```python
from build123d import *

# Parameters (mm, degrees)
F0_R     = 1.7272
F0_R_2   = 3.2639
F0_R_3   = 2.4003
F1_DEPTH = 99.06
F2_DEPTH = 88.9
F3_DEPTH = 25.4
F4_DEPTH = 99.061
F5_R     = 1.7272
F6_DEPTH = 5.08
F7_DEPTH = 15.24
F5_R_2   = 1.5875
F8_DEPTH = 19.6383854826


with BuildPart() as f1:
    # F0 (on Front) → F1 (new body)
    with BuildSketch(Plane.XZ):
        with BuildLine():
            Line((-9.525, -12.7), (9.525, -12.7))
            ThreePointArc((9.525, -12.7), (0, 15.875), (-9.525, -12.7))
        make_face()
        with Locations((-9.525, -1.905)):
            Circle(F0_R, mode=Mode.SUBTRACT)
        with Locations((9.525, -1.905)):
            Circle(F0_R, mode=Mode.SUBTRACT)
        with Locations((0, 8.7377419695)):
            Circle(F0_R_2, mode=Mode.SUBTRACT)
        with Locations((0, 8.7377419695)):
            Circle(F0_R_2)
        with Locations((0, 8.7377419695)):
            Circle(F0_R_3, mode=Mode.SUBTRACT)
        with Locations((-9.525, -1.905)):
            Circle(F0_R)
        with Locations((9.525, -1.905)):
            Circle(F0_R)
    extrude(amount=-F1_DEPTH)

    # F0 (on Front) → F2 (cut, through all)
    with BuildSketch(Plane.XZ):
        with Locations((0, 8.7377419695)):
            Circle(F0_R_2)
        with Locations((0, 8.7377419695)):
            Circle(F0_R_3, mode=Mode.SUBTRACT)
    extrude(amount=-F2_DEPTH, mode=Mode.SUBTRACT)

    # F0 (on Front) → F3 (cut)
    with BuildSketch(Plane.XZ):
        with Locations((-9.525, -1.905)):
            Circle(F0_R)
        with Locations((9.525, -1.905)):
            Circle(F0_R)
    extrude(amount=-F3_DEPTH, mode=Mode.SUBTRACT)

    # F0 (on Front) → F4 (cut, through all)
    with BuildSketch(Plane.XZ):
        with Locations((0, 8.7377419695)):
            Circle(F0_R_3)
    extrude(amount=-F4_DEPTH, mode=Mode.SUBTRACT)

    # F5 (on face) → F6 (cut)
    with BuildSketch(Plane(origin=(0, 0, -12.7), x_dir=(1, 0, 0), z_dir=(0, 0, -1))):
        with BuildLine():
            Line((-9.525, -84.5499397641), (-9.525, -8.5156602359))
            ThreePointArc((-9.525, -8.5156602359), (-17.1876576863, -11.3104638467), (-24.1058971733, -15.6307893484))
            Line((-24.1058971733, -15.6307893484), (-24.1058971733, -77.4348106516))
            ThreePointArc((-24.1058971733, -77.4348106516), (-17.1876576863, -81.7551361533), (-9.525, -84.5499397641))
        make_face()
        with BuildLine():
            Line((9.525, -84.5499397641), (9.525, -8.5156602359))
            ThreePointArc((9.525, -8.5156602359), (0, -7.3406), (-9.525, -8.5156602359))
            Line((-9.525, -8.5156602359), (-9.525, -84.5499397641))
            ThreePointArc((-9.525, -84.5499397641), (0, -85.725), (9.525, -84.5499397641))
        make_face()
        with Locations((0, -46.5328)):
            Circle(F5_R, mode=Mode.SUBTRACT)
        with BuildLine():
            ThreePointArc((19.2613247782, -12.4002655405), (14.5236243119, -10.1309748028), (9.525, -8.5156602359))
            Line((9.525, -8.5156602359), (9.525, -84.5499397641))
            ThreePointArc((9.525, -84.5499397641), (14.5236243119, -82.9346251972), (19.2613247782, -80.6653344595))
            Line((19.2613247782, -80.6653344595), (19.2613247782, -12.4002655405))
        make_face()
        with BuildLine():
            ThreePointArc((19.2613247782, -87.8013515693), (14.4855288925, -89.7098938525), (9.525, -91.067801469))
            Line((9.525, -91.067801469), (9.525, -99.06))
            Line((9.525, -99.06), (19.2613247782, -99.06))
            Line((19.2613247782, -99.06), (19.2613247782, -87.8013515693))
        make_face()
        with BuildLine():
            Line((9.525, -99.06), (9.525, -91.067801469))
            ThreePointArc((9.525, -91.067801469), (0, -92.075), (-9.525, -91.067801469))
            Line((-9.525, -91.067801469), (-9.525, -99.06))
            Line((-9.525, -99.06), (9.525, -99.06))
        make_face()
        with BuildLine():
            Line((-9.525, -99.06), (-9.525, -91.067801469))
            ThreePointArc((-9.525, -91.067801469), (-17.0718789618, -88.7541563206), (-24.1058971733, -85.1721284402))
            Line((-24.1058971733, -85.1721284402), (-24.1058971733, -99.06))
            Line((-24.1058971733, -99.06), (-9.525, -99.06))
        make_face()
        with BuildLine():
            Line((9.525, 0), (9.525, -1.997798531))
            ThreePointArc((9.525, -1.997798531), (14.4855288925, -3.3557061475), (19.2613247782, -5.2642484307))
            Line((19.2613247782, -5.2642484307), (19.2613247782, 0))
            Line((19.2613247782, 0), (9.525, 0))
        make_face()
        with BuildLine():
            ThreePointArc((-9.525, -1.997798531), (0, -0.9906), (9.525, -1.997798531))
            Line((9.525, -1.997798531), (9.525, 0))
            Line((9.525, 0), (-9.525, 0))
            Line((-9.525, 0), (-9.525, -1.997798531))
        make_face()
        with BuildLine():
            ThreePointArc((-24.1058971733, -7.8934715598), (-17.0718789618, -4.3114436794), (-9.525, -1.997798531))
            Line((-9.525, -1.997798531), (-9.525, 0))
            Line((-9.525, 0), (-24.1058971733, 0))
            Line((-24.1058971733, 0), (-24.1058971733, -7.8934715598))
        make_face()
    extrude(amount=-F6_DEPTH, mode=Mode.SUBTRACT)

    # F5 (on face) → F7 (cut)
    with BuildSketch(Plane(origin=(0, 0, -12.7), x_dir=(1, 0, 0), z_dir=(0, 0, -1))):
        with Locations((0, -46.5328)):
            Circle(F5_R)
    extrude(amount=-F7_DEPTH, mode=Mode.SUBTRACT)

    # F5 (on face) → F8 (cut, through all)
    with BuildSketch(Plane(origin=(0, 0, -12.7), x_dir=(1, 0, 0), z_dir=(0, 0, -1))):
        with Locations((0, -88.9)):
            Circle(F5_R_2)
        with Locations((0, -4.1656)):
            Circle(F5_R_2)
    extrude(amount=-F8_DEPTH, mode=Mode.SUBTRACT)


solid = f1.part
```
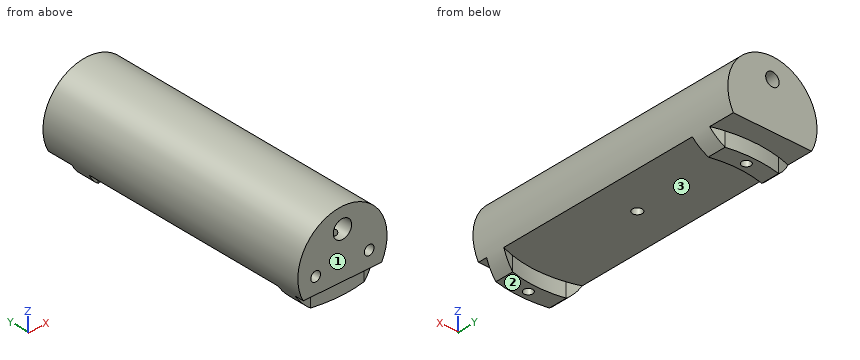
Geometry: final body of the model. Coordinates: model frame, mm. Face numbers are marked on the shaded views. Round coordinates to 2 decimals unless told otherwise and drop trailing zeros. Order: outer loops, then holes, each group sorted by start corner. A loop starts at its lowest first (then second) coordinate and runs counter-clockwise, first axis right, second up. Notation, with made-up numbers: (-27.75, 47.25) - (-18.75, 47.25) arc R7 ccw to (-18.75, 54.25) - close; hole circle Ø6 at (69, 53.25). An arc over 180 degrees is marked (long way). Write item = value, one per line. Start each with the question number.
Q1. Pull-direction query (Y, two-part tool) for the marked faces 1, 2 and 3; classes: +Y half, -Y half, draft (parallel to the pull), parting line (faces both ways), or undercut.
Q2. Cut plane A-A on x = 0. Give the number of separate pieces and of enclosed holes in the cut face, and give its area (3 significant figures).
Q3. Ray query, line 1 (Y direction, x = 0, z = -1); line 2 (Z direction, x = 0, y = 95.5) (3 decimals); line 3 (Z direction, x = 0, y = 48.5) (3 decimals). Return the intervals inside material, ascending. Write a range as from..to.
Q4. Pin query (flat end, axial travel): pin 1 (1.9 mm diameter, centred on x = 0, y = 88.9, fed in from -Z); pin 2 (6 mm diameter, centred on y = 34.5, z = 8.5, fed in from -X); pin 3 (12 mm diameter, centred on x = -12, y = 83, fed in from -Z); pin 4 (7.5 mm diameter, centred on x = 2, y = 96.5, fed in from -Z). Return the tip coordinate at first contact, or that it passes through.
Q5. Cut plane B-B on x = 13. Return the cut outline in (y, z), and give its area (3 significant figures).
Q6. Cut plane C-C on y = 78.5. Return the cut outline in (x, z) (3 decimals), and give its area (3 significant figures).
Outcome:
q1.face_1 = -Y half
q1.face_2 = draft
q1.face_3 = undercut
q2.separate_pieces = 4
q2.enclosed_holes = 0
q2.area = 1,610 mm^2
q3.line_1 = 0..2.58, 5.75..44.81, 48.26..87.31, 90.49..99.06
q3.line_2 = -7.62..6.337, 11.138..15.875
q3.line_3 = -7.62..5.474, 12.002..15.875
q4.pin_1 = 10.94
q4.pin_2 = -14.89
q4.pin_3 = -12.7
q4.pin_4 = -7.62
q5.outline = (0, -7.62) - (2.89, -7.62) - (2.89, -9.11) - (9.56, -9.11) - (9.56, -7.62) - (83.51, -7.62) - (83.51, -9.11) - (90.18, -9.11) - (90.18, -7.62) - (99.06, -7.62) - (99.06, 9.11) - (0, 9.11) - close
q5.area = 1,680 mm^2
q6.outline = (-13.927, -7.62) - (13.927, -7.62) arc R15.875 ccw (long way) to start; hole circle Ø6.528 at (0, 8.738)
q6.area = 595 mm^2
